Read the model definition and answer for the solid it produces. Units are mm, in the model's axes. Round coordinates to 2 decimals unless told otherwise and drop trailing zeros. One line per item, written item: value. Start each with the question number.
1. The mould has two halves that part along Z. Classify faces 1 (the face through (-113, 21, 2.5)), 2 (the face through (0, -3, 0)), 3 (the face through (-113, 21, -2.5)): released by +Z, released by -Z, zero draft, split by the parting line, or undercut.
2. Consider line 1 (Y direction, x = -127.5, z = 1.55); line 2 (X direction, y = 74.5, z = 2.15); line 3 (Y direction, x = -133, z = 1.35). Determine where each line is inside the solid, lowest interval first.
3. A flat-ended cylindrical pin translates along its axis: pin 1 Ø1.5 at (x, z) = (-121.5, 1.5) entering from +Y. Find the tip coordinate at first contact, or state that the pin passes through.
from build123d import *

# Parameters (mm, degrees)
BOSS_EXTRUDE1_DEPTH = 2.5


with BuildPart() as part:
    # Sketch1 → Boss-Extrude1 (new, symmetric)
    with BuildSketch(Plane.XY):
        with BuildLine():
            Line((-138.606439558, 88.2396), (-154.481439558, 88.2396))
            Line((-154.481439558, 88.2396), (-154.481439558, -6.35))
            Line((-154.481439558, -6.35), (0, -6.35))
            Line((0, -6.35), (0, 0))
            add(Edge.make_bspline(
                [(-138.606439558, 88.2396), (-138.606439558, 88.206480064), (-138.604893224, 88.134332137), (-138.597757085, 87.982040168), (-138.584504009, 87.767973581), (-138.563362589, 87.511833211), (-138.514302662, 87.023426652), (-138.425196169, 86.336581908), (-138.262733573, 85.340165391), (-137.997774346, 84.039042844), (-137.543893872, 82.163940465), (-136.709143666, 79.332808223), (-135.381511976, 75.692405853), (-133.427089014, 71.311625777), (-130.978665346, 66.686011286), (-128.248792738, 62.200876138), (-125.278396767, 57.871801388), (-121.922980854, 53.47598485), (-117.499907722, 48.25477976), (-111.846477366, 42.372548658), (-104.806706424, 36.032698765), (-96.481239759, 29.625824358), (-87.711829988, 23.843138375), (-78.562226684, 18.684637722), (-69.088219119, 14.150320925), (-59.340712588, 10.240190432), (-49.365347684, 6.954244107), (-41.111501611, 4.791563651), (-34.694119901, 3.420549472), (-30.177735786, 2.597379945), (-27.586849558, 2.166008761), (-24.349433278, 1.675559443), (-20.435573897, 1.165043535), (-15.888225625, 0.68322541), (-11.278370624, 0.337947753), (-7.392012303, 0.139524343), (-4.35262006, 0.048647043), (-2.477110072, 0.012428268), (-0.93320285, 0.001817838), (-0.315317676, 0), (0, 0)],
                knots=[0, 0, 0, 0, 0, 0.000750682, 0.001501364, 0.003002728, 0.004504092, 0.006005456, 0.011632897, 0.017260339, 0.025307868, 0.033355398, 0.051377592, 0.078047856, 0.105080676, 0.132113154, 0.15914583, 0.186178382, 0.213211084, 0.24601624, 0.3000815, 0.354146872, 0.408211991, 0.462277325, 0.516342503, 0.570407831, 0.624473028, 0.67853828, 0.732603517, 0.746119838, 0.759636158, 0.773152478, 0.786668798, 0.813701417, 0.840734035, 0.867766658, 0.88128297, 0.894799281, 0.901946134, 0.909092986, 0.909092986, 0.909092986, 0.909092986, 0.909092986], degree=4))
        make_face()
    extrude(amount=BOSS_EXTRUDE1_DEPTH, both=True)


solid = part.part
Answer:
1. face 1: released by +Z
1. face 2: zero draft
1. face 3: released by -Z
2. line 1: -6.35 to 61.17
2. line 2: -154.48 to -134.81
2. line 3: -6.35 to 70.61
3. pin 1: y = 53.98
